Check sheet for the modelled part. Datum: model origin and axes. Units: mm. Face numbers are marked on the shaded views. A direction names the side the tool comes from. Round coordinates to 2 decimals unless told otherwise and drop trailing zeros. Loops run counter-clockwise (first coordinate to the right, second up) from the corner with the lowest first, then second, coordinate; pieces in that order, holes last. Notation, with made-up numbers: (79.25, 24) -> (131.25, 24) arc R17 cw to (131.25, 33) -> close; hole circle Ø1 at (21.25, -9). An arc over 180 degrees is marked (long way). One line per item, written item: value. Start each with the question number.
1. Material ranges on L1, parallel to Y at x = 17, z = 3.5, recorded low to high.
2. Set-up check for the marked faces 5 and 6: record each of +Z, -Z, +X, -X, +Y, -Y from which the full face is reachable in a straight line by a thin tool's end or side.
3. Go/stop test with a flat-tipped pin: pin 1 (0.7 mm diameter, centred on x = 42, z = 4.5, fed in from +Y). Record where the tip stops, or that it passes through.
4. Cross-section at D-D on x = 25. Record the cut outline in (y, z).
5. Cross-section at C-C on x = 35.5. Record the cut outline in (y, z), then the cut area to 3 significant figures.
6. Release check for a two-part mould opening along X. For the marked faces 1, 2, 3 and 4 record: +X half, -X half, draft (parallel to the pull), parting line (faces both ways), or undercut.
7. Cross-section at A-A on y = 8.25. Count the separate pieces of the cut face and the enclosed holes in it, then the cut area to 3 significant figures.
from build123d import *

# Parameters (mm, degrees)
SKETCH_1_W             = 50
SKETCH_1_H             = 10
EXTRUDE_1_DEPTH        = 10
CUT_EXTRUDE_1_DEPTH    = 52.961524227
PATTERN_LINEAR_1_COUNT = 7
PATTERN_LINEAR_1_PITCH = 6.28


with BuildPart() as part:
    # 草图1 → 凸台-拉伸1 (new body)
    with BuildSketch(Plane.XY):
        with Locations((25, 5)):
            Rectangle(SKETCH_1_W, SKETCH_1_H)
    extrude(amount=EXTRUDE_1_DEPTH)

    # 草图2 → 切除-拉伸1 (cut, through all)
    with BuildSketch(Plane.XY.offset(10)):
        Polygon((2, 10), (3.637866054, 5.5), (4.959614883, 5.5), (6.597480937, 10), align=None)
    cut_extrude_1 = extrude(amount=-CUT_EXTRUDE_1_DEPTH, mode=Mode.SUBTRACT)

    # 阵列(线性)1: 切除-拉伸1 ×7
    with Locations(*[(i * PATTERN_LINEAR_1_PITCH, 0, 0) for i in range(1, PATTERN_LINEAR_1_COUNT)]):
        add(cut_extrude_1, mode=Mode.SUBTRACT)


solid = part.part
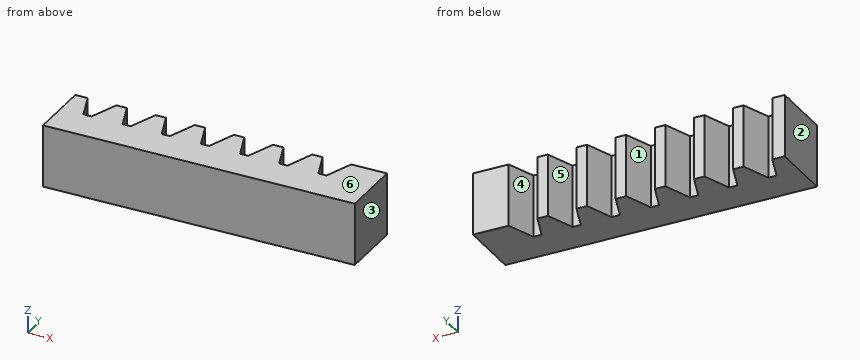
Taken from the geometry:
1. L1: y = 0 to 5.5
2. face 5: +Z, -Z, +Y
2. face 6: +Z, +X, -X, +Y, -Y
3. pin 1: stops at y = 5.5
4. outline: (0, 0) -> (8.8, 0) -> (8.8, 10) -> (0, 10) -> close
5. outline: (0, 0) -> (5.5, 0) -> (5.5, 10) -> (0, 10) -> close
5. area: 55.0 mm2
6. face 1: undercut
6. face 2: -X half
6. face 3: +X half
6. face 4: undercut
7. separate pieces: 8
7. enclosed holes: 0
7. area: 267 mm2
